For this review, take the finished solid that the model builds, in its own axes (mm). Face numbers are marked on the shaded views. A direction names the side the tool comes from. Give positions to 0.01 mm unless a question says otherwise; leave off trailing zeros. Loops run counter-clockwise (first coordinate to the right, second up) from the corner with the lowest first, then second, coordinate; pieces in that order, holes last.
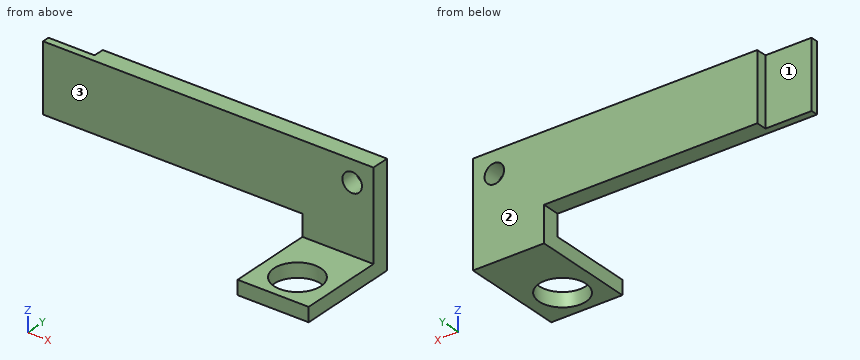
```python
from build123d import *

# Parameters (mm, degrees)
SKETCH001_W   = 20
SKETCH001_H   = 4
PAD001_DEPTH  = 29
SKETCH002_R   = 6.6
HOLE_DEPTH    = 4.001001
SKETCH004_W   = 13
SKETCH004_H   = 3
PAD002_DEPTH  = 19
PAD_DEPTH     = 5
SKETCH003_R   = 2.75
HOLE001_DEPTH = 5.001


with BuildPart() as body001:
    # Sketch001 (on Face1 of CopyPad) → Pad001 (new body)
    with BuildSketch(Plane(origin=(0, 0, 0), x_dir=(-1, 0, 0), z_dir=(0, 1, 0))):
        with Locations((-102, -115)):
            Rectangle(SKETCH001_W, SKETCH001_H)
    extrude(amount=-PAD001_DEPTH)

    # Sketch002 (on Face3 of Pad001) → Hole (cut, through all)
    with BuildSketch(Plane(origin=(0, 3e-06, -117), x_dir=(1, 0, 0), z_dir=(0, 0, -1))):
        with Locations((102, 20)):
            Circle(SKETCH002_R)
    extrude(amount=-HOLE_DEPTH, mode=Mode.SUBTRACT)


with BuildPart() as body002:
    # Sketch004 (on Face1 of CopyHole001) → Pad002 (new body)
    with BuildSketch(Plane(origin=(0, 0, -107), x_dir=(1, 0, 0), z_dir=(0, 0, -1))):
        with Locations((25.5, 39.5)):
            Rectangle(SKETCH004_W, SKETCH004_H)
    extrude(amount=-PAD002_DEPTH)


with BuildPart() as body002_1:
    # Body002 placement: moved
    add(body002.part.moved(Location((0, 38, 0))))


with BuildPart() as body:
    # Sketch → Pad (new body)
    with BuildSketch(Plane.XZ):
        Polygon((19, -88), (112, -88), (112, -117), (92, -117), (92, -107), (19, -107), align=None)
    extrude(amount=PAD_DEPTH)

    # Sketch003 (on Face8 of Pad) → Hole001 (cut, through all)
    with BuildSketch(Plane.XZ.offset(5)):
        with Locations((106, -94)):
            Circle(SKETCH003_R)
    extrude(amount=-HOLE001_DEPTH, mode=Mode.SUBTRACT)

    # Boolean: union Body001
    add(body001.part)

    # Boolean001: cut Body002
    add(body002_1.part, mode=Mode.SUBTRACT)


solid = body.part
```
Q1. For pin 1 Ø7.5 at (x, z) = (66, -98) entering from -Y; pin 2 Ø12 at (x, z) = (61.5, -106.5) entering from +Y; pin 3 Ø1.5 at (x, y) = (45, -1.5) entering from -Z; pin 4 Ø5 at (y, z) = (-21.5, -112) entering from -X, all flat-tipped, find the tip position at first contact; note any pin that passes through.
Answers:
pin 1: stops at y = -5
pin 2: stops at y = 0
pin 3: stops at z = -107
pin 4: stops at x = 92
Q2. Consider section A-A on z = -94. Give the boundary of the cut face in (x, y).
Answers:
outline: (19, -5) - (103.25, -5) - (103.25, 0) - (32, 0) - (32, -3) - (19, -3) - close; (108.75, -5) - (112, -5) - (112, 0) - (108.75, 0) - close
Q3. For probe 1 along Y at (x, z) = (102, -114.85); probe 2 along Z at (x, y) = (106, -3.55); probe 3 along Y at (x, z) = (75.5, -94.75), list the stretches that pass through material, from the lowest coordinate up.
Answers:
probe 1: y = -29 to -26.6, -13.4 to 0
probe 2: z = -117 to -96.75, -91.25 to -88
probe 3: y = -5 to 0
Q4. Consider section B-B on x = 102. Give the boundary of the cut face in (y, z), plus the area to 3 significant figures.
Answers:
outline: (-29, -117) - (-26.6, -117) - (-26.6, -113) - (-29, -113) - close; (-13.4, -117) - (0, -117) - (0, -88) - (-5, -88) - (-5, -113) - (-13.4, -113) - close
area: 188 mm2
Q5. Consider section D-D on z = -101. Give the boundary of the cut face in (x, y).
Answers:
outline: (19, -5) - (112, -5) - (112, 0) - (32, 0) - (32, -3) - (19, -3) - close
Q6. Machinability: for the marked faces 1, 2 and 3, which of the approach directions +Z, -Z, +X, -X, +Y, -Y give a long, thin tool a straight path to every point of the face, cutting with its end or side? Answer none if there is none.
Answers:
face 1: +Z, -Z, -X, +Y
face 2: +Z, -Z, +X, -X, +Y
face 3: +Z, +X, -X, -Y
Q7. Consider section C-C on y = -21.25. Give the boundary of the cut face in (x, z), plus the area to 3 significant figures.
Answers:
outline: (92, -117) - (95.52, -117) - (95.52, -113) - (92, -113) - close; (108.48, -117) - (112, -117) - (112, -113) - (108.48, -113) - close
area: 28.2 mm2
